from build123d import *

# Parameters (mm, degrees)
BOSS_EXTRUDE1_DEPTH      = 2.6
BOSS_EXTRUDE1_DEPTH_BACK = 6
FILLET1_R                = 20
CUT_EXTRUDE1_DEPTH       = 5
SKETCH5_R                = 2
CUT_EXTRUDE2_DEPTH       = 20
FILLET3_R                = 1
CIRPATTERN1_COUNT        = 3
SKETCH6_R                = 2.75
CUT_EXTRUDE3_DEPTH       = 56.475677209
BOSS_EXTRUDE2_DEPTH      = 4
SKETCH8_R                = 2.1
CUT_EXTRUDE4_DEPTH       = 76.353770721
CHAMFER1_SIZE            = 2.5
SKETCH9_R                = 1.5
CUT_EXTRUDE5_DEPTH       = 76.353770721
BOSS_EXTRUDE3_START      = -2.35
BOSS_EXTRUDE3_DEPTH      = 2.35
BOSS_EXTRUDE4_DEPTH      = 2.35
SKETCH12_R               = 2.8
CUT_EXTRUDE6_DEPTH       = 2.35
FILLET4_R                = 10


with BuildPart() as part:
    # Sketch3 → Boss-Extrude1 (new, two sides: drawn at the far end of the back side and taken through both)
    with BuildSketch(Plane.XY.offset(-BOSS_EXTRUDE1_DEPTH_BACK)):
        Polygon((-25, 39), (25, 39), (25, -3.511595657), (38.504425224, -11.308379196), (33.774990748, -19.5), (29.045556271, -27.691620804), (-29.045556271, -27.691620804), (-33.774990748, -19.5), (-38.504425224, -11.308379196), (-25, -3.511595657), align=None)
    extrude(amount=BOSS_EXTRUDE1_DEPTH + BOSS_EXTRUDE1_DEPTH_BACK)

    # Fillet1
    fillet1_edges = [part.edges().sort_by_distance(p)[0] for p in [
        (25, -3.511595657, -1.7),
        (-25, -3.511595657, -1.7),
    ]]
    fillet(fillet1_edges, radius=FILLET1_R)

    # Sketch4 → Cut-Extrude1 (cut, symmetric)
    with BuildSketch(Plane(origin=(0, 30, 0), x_dir=(1, 0, 0), z_dir=(0, 1, 0))):
        Polygon((5.114783638, 0.485216362), (-5.114783638, 0.485216362), (-6, -0.4), (-6, -2.6), (6, -2.6), (6, -0.4), align=None)
    cut_extrude1 = extrude(amount=CUT_EXTRUDE1_DEPTH, both=True, mode=Mode.SUBTRACT)

    # Sketch5 → Cut-Extrude2 (cut)
    with BuildSketch(Plane(origin=(0, 39, 0), x_dir=(1, 0, 0), z_dir=(0, 1, 0))):
        with Locations(Location((-4.458868953, 0, 0), (0, 0, 180))):
            Circle(SKETCH5_R)
        with Locations(Location((4.458868953, 0, 0), (0, 0, 180))):
            Circle(SKETCH5_R)
    cut_extrude2 = extrude(amount=-CUT_EXTRUDE2_DEPTH, mode=Mode.SUBTRACT)

    # Fillet3
    fillet3_edges = [part.edges().sort_by_distance(p)[0] for p in [
        (-6, 30, 2.6),
        (6, 30, 2.6),
    ]]
    fillet(fillet3_edges, radius=FILLET3_R)

    # CirPattern1: Cut-Extrude1, Cut-Extrude2 ×3 about axis
    cirpattern1_axis = Axis((0, 0, 0), (0, 0, 1))
    add([cut_extrude1.rotate(cirpattern1_axis, i * 360 / CIRPATTERN1_COUNT) for i in range(1, CIRPATTERN1_COUNT)], mode=Mode.SUBTRACT)
    add([cut_extrude2.rotate(cirpattern1_axis, i * 360 / CIRPATTERN1_COUNT) for i in range(1, CIRPATTERN1_COUNT)], mode=Mode.SUBTRACT)

    # Sketch6 → Cut-Extrude3 (cut, through all)
    with BuildSketch(Plane.XY.offset(2.6)):
        Circle(SKETCH6_R)
    extrude(amount=-CUT_EXTRUDE3_DEPTH, mode=Mode.SUBTRACT)

    # Sketch7 → Boss-Extrude2 (add)
    with BuildSketch(Plane(origin=(0, 0, -6), x_dir=(-1, 0, 0), z_dir=(0, 0, -1))):
        with BuildLine():
            Line((-25, 39), (25, 39))
            Line((25, 39), (25, 54))
            Line((25, 54), (2.36629775, 63.713677082))
            ThreePointArc((2.36629775, 63.713677082), (0, 64.2), (-2.36629775, 63.713677082))
            Line((-2.36629775, 63.713677082), (-25, 54))
            Line((-25, 54), (-25, 39))
        make_face()
    extrude(amount=-BOSS_EXTRUDE2_DEPTH)

    # Sketch8 → Cut-Extrude4 (cut, through all)
    with BuildSketch(Plane.XY.offset(2.6)):
        with Locations((-19, 13.2)):
            Circle(SKETCH8_R)
        with Locations((19, 13.2)):
            Circle(SKETCH8_R)
        with Locations((0, 58.2)):
            Circle(SKETCH8_R)
    extrude(amount=-CUT_EXTRUDE4_DEPTH, mode=Mode.SUBTRACT)

    # Chamfer1
    chamfer1_edges = [part.edges().sort_by_distance(p)[0] for p in [
        (-21.1, 13.2, 2.6),
        (16.9, 13.2, 2.6),
        (-2.1, 58.2, -2),
    ]]
    chamfer(chamfer1_edges, length=CHAMFER1_SIZE)

    # Sketch9 → Cut-Extrude5 (cut, through all)
    with BuildSketch(Plane(origin=(0, 0, -6), x_dir=(-1, 0, 0), z_dir=(0, 0, -1))):
        with Locations((7.5, -21.041620804)):
            Circle(SKETCH9_R)
        with Locations((-2, -21.041620804)):
            Circle(SKETCH9_R)
    extrude(amount=-CUT_EXTRUDE5_DEPTH, mode=Mode.SUBTRACT)

    # Sketch10 → Boss-Extrude3 (add)
    with BuildSketch(Plane(origin=(0, 0, -6), x_dir=(-1, 0, 0), z_dir=(0, 0, -1)).offset(BOSS_EXTRUDE3_START)):
        with BuildLine():
            Line((25, 54), (38.504425224, 48.204323078))
            Line((38.504425224, 48.204323078), (38.504425224, -11.308379196))
            Line((38.504425224, -11.308379196), (35, -9.285098349))
            ThreePointArc((35, -9.285098349), (27.679491924, -1.964590274), (25, 8.035409726))
            Line((25, 8.035409726), (25, 54))
        make_face()
    extrude(amount=BOSS_EXTRUDE3_DEPTH)

    # Sketch11 → Boss-Extrude4 (add)
    with BuildSketch(Plane(origin=(0, 0, -6), x_dir=(-1, 0, 0), z_dir=(0, 0, -1))):
        with BuildLine():
            Line((-38.504425224, -11.308379196), (-38.504425224, 64.2))
            Line((-38.504425224, 64.2), (0, 64.2))
            ThreePointArc((0, 64.2), (-1.20787779, 64.077161836), (-2.36629775, 63.713677082))
            Line((-2.36629775, 63.713677082), (-25, 54))
            Line((-25, 54), (-25, 8.035409726))
            ThreePointArc((-25, 8.035409726), (-27.679491924, -1.964590274), (-35, -9.285098349))
            Line((-35, -9.285098349), (-38.504425224, -11.308379196))
        make_face()
    extrude(amount=-BOSS_EXTRUDE4_DEPTH)

    # Sketch12 → Cut-Extrude6 (cut)
    with BuildSketch(Plane.XY.offset(-3.65)):
        with Locations((-31, 39.8275)):
            Circle(SKETCH12_R)
        with Locations((31, 50.8275)):
            Circle(SKETCH12_R)
        with Locations((-31, 21.0775)):
            Circle(SKETCH12_R)
        with Locations((31, 32.0775)):
            Circle(SKETCH12_R)
    extrude(amount=-CUT_EXTRUDE6_DEPTH, mode=Mode.SUBTRACT)

    # Fillet4
    fillet4_edges = [part.edges().sort_by_distance(p)[0] for p in [
        (38.504425224, 64.2, -4.825),
    ]]
    fillet(fillet4_edges, radius=FILLET4_R)


solid = part.part
Here's how the part is built. I have some questions about the finished solid (model axes, mm). A direction names the side the tool comes from. Give positions to 0.01 mm unless a question says otherwise; leave off trailing zeros. Loops run counter-clockwise (first coordinate to the right, second up) from the corner with the lowest first, then second, coordinate; pieces in that order, holes last. Notation, with made-up numbers: (36, 58.5) -> (76, 58.5) arc R19 cw to (76, 86.5) -> close; hole circle Ø7 at (18.25, 17.25). An arc over 180 degrees is marked (long way). Answer as a JSON object with one key per item and string values. Group by question number.
Item 1: I need wall thicknesses on L1, parallel to Y at x = 0, z = 0.25; L2, parallel to X at y = 13.5, z = -5.5; L3, parallel to X at y = -12.5, z = 1.5. Which ranges of each line are inside material? Lowest first, please.
Item 2: Imagine slicing it at C-C on y = 0. Write out the boundary of the cut face in (x, z).
Item 3: Imagine slicing it at B-B on x = 11.5. Write out the boundary of the cut face in (y, z), then the cut area to 3 significant figures.
Item 4: Thinking about a two-plate mould opening in X: for faces 1 (the flat face through (36.728, -10.283, -0.569)), 2 (the flat face through (28, 32, -3.65)), 3 (the flat face through (-18.7, -5.61, 0.03)), 4 (the flat face through (-36.777, -10.311, -0.569)), which applies, pulls with the +X half, pulls with the -X half, needs draft (parallel to the pull), parting line crosses it, or undercut?
Item 5: On a 3-axis mill with a long thin cutter (end or side, diameter ignored), from which of +Z, -Z, +X, -X, +Y, -Y can I reach the whole of each face in a straight line? I mean faces 5 (the cylindrical face through (-0.574, 64.173, -3.584)), 6 (the cylindrical face through (-5.382, 29.14, -1.774)), 7 (the flat face through (-14.239, -13.337, 0.028)). Say none if no direction works.
Item 6: Imagine slicing it at A-A on y = 33.5. Write out the boundary of the cut face in (x, z), then the cut area to 3 significant figures.
Item 7: Will these pins go through, and if not, where does the flat tip stop? pin 1 (2 mm diameter, centred on y = 36, z = 1, fed in from +X); pin 2 (6 mm diameter, centred on x = 27, y = 46.5, fed in from +Z); pin 3 (4.5 mm diameter, centred on x = 0, y = 0, fed in from +Z); pin 4 (5.5 mm diameter, centred on x = 0, y = 58.2, fed in from +Z).
Answer list:
{
 "1": {"L1": "y = -27.69 to -2.75, 2.75 to 25, 35 to 39", "L2": "x = -38.5 to -21.08, -16.92 to 16.92, 21.08 to 38.5", "L3": "x = -37.82 to -33.21, -21.65 to -15.38, -14.72 to 14.72, 15.38 to 21.65, 33.21 to 37.82"},
 "2": {"outline": "(-38.5, -6) -> (-2.75, -6) -> (-2.75, 2.6) -> (-26.69, 2.6) -> (-26.69, -3.65) -> (-38.5, -3.65) -> close; (2.75, -6) -> (38.5, -6) -> (38.5, -3.65) -> (26.69, -3.65) -> (26.69, 2.6) -> (2.75, 2.6) -> close"},
 "3": {"outline": "(-27.69, -6) -> (64.2, -6) -> (64.2, -3.65) -> (59.79, -3.65) -> (59.79, -2) -> (39, -2) -> (39, 2.6) -> (-27.69, 2.6) -> close", "area": "667 mm2"},
 "4": {"face 1": "pulls with the +X half", "face 2": "needs draft", "face 3": "undercut", "face 4": "pulls with the -X half"},
 "5": {"face 5": "+Z, +Y", "face 6": "+Y", "face 7": "none"},
 "6": {"outline": "(-38.5, -6) -> (28.59, -6) -> (28.59, -3.65) -> (25, -3.65) -> (25, 2.6) -> (7, 2.6) arc R1 ccw to (6, 1.6) -> (6, 1.27) arc R2 cw (long way) to (2.52, -0.49) -> (-2.52, -0.49) arc R2 cw (long way) to (-6, 1.27) -> (-6, 1.6) arc R1 ccw to (-7, 2.6) -> (-25, 2.6) -> (-25, -3.65) -> (-38.5, -3.65) -> close; (33.41, -6) -> (38.5, -6) -> (38.5, -3.65) -> (33.41, -3.65) -> close", "area": "435 mm2"},
 "7": {"pin 1": "stops at x = 25", "pin 2": "stops at z = -2", "pin 3": "passes through", "pin 4": "stops at z = -3.85"}
}
